The model under review builds one solid part; all positions refer to its coordinate system, in mm. A direction names the side the tool comes from. Give positions to 0.01 mm unless a question says otherwise; leave off trailing zeros. Write each question's results on one line, items separated by ' | '. Start each with the question number.
Q1. Machinability: for faces 5 (the face through (321, 11, -652.571)), 6 (the face through (321, 4, -649.396)), 7 (the face through (321, 24, -652.571)), 8 (the face through (318.96, 7, -681)), 9 (the face through (321, -0.32, -651)), which of the approach directions +Z, -Z, +X, -X, +Y, -Y give a long, thin tool a straight path to every point of the face, cutting with its end or side? Answer none if there is none.
Q2. Insertion check: pin 1 Ø1.6 at (x, z) = (320.5, -651.5) entering from +Y; pin 2 Ø1.1 at (x, y) = (321, 24) entering from +Z; pin 3 Ø1 at (x, z) = (320, -651) entering from -Y. Each pin has a flat end and moves straight along its axis. Give the tip position at first contact, or say it passes through.
Q3. Wall thickness on L1, parallel to Y at x = 320.15, z = -671; L2, parallel to Y at x = 320.15, z = -740: over which ranges is each line inside the solid? List them lowest first. Write a range as [from, to].
Q4. Mouldability with a two-part tool opening along Y and no side actions: class faces 1 (the face through (321, 13.65, -651)), 2 (the face through (321, -9, -764.915)), 3 (the face through (321, 22.54, -651)), 4 (the face through (321, 8.57, -651)) as released by +Y, released by -Y, zero draft, split by the parting line, or undercut.
from build123d import *

# Parameters (mm, degrees)
BOSS_EXTRUDE1_DEPTH = 3.175
CUT_EXTRUDE1_DEPTH  = 3.175
SKETCH3_W           = 3.175
SKETCH3_H           = 8.89
BOSS_EXTRUDE3_DEPTH = 3.175


with BuildPart() as part:
    # Sketch1 → Boss-Extrude1 (new body)
    with BuildSketch(Plane(origin=(322.1355, 0, 0), x_dir=(0, 0, -1), z_dir=(1, 0, 0))):
        with BuildLine():
            Line((652.571489798, 25.444691841), (652.571489798, -2.239853871))
            add(Edge.make_bspline(
                [(652.571489798, -2.239853871), (659.535508053, -2.166526792), (666.500386762, -2.172540218), (679.343468905, -2.343824355), (685.222739923, -2.485063976), (696.978954297, -2.909271923), (702.85456416, -3.191578316), (714.592323323, -3.919191383), (720.455505411, -4.364295636), (729.239801176, -5.181453913), (732.167256327, -5.479520855), (738.010202726, -6.135780349), (740.925935315, -6.494041299), (749.652482821, -7.677212837), (755.443511526, -8.605976907), (762.435970423, -9.996546686), (763.676377356, -10.253772029), (764.914772229, -10.521558234)],
                knots=[0.775497337, 0.775497337, 0.775497337, 0.775497337, 0.8125, 0.8125, 0.84375, 0.84375, 0.875, 0.875, 0.90625, 0.90625, 0.921875, 0.921875, 0.9375, 0.9375, 0.96875, 0.96875, 0.975501731, 0.975501731, 0.975501731, 0.975501731], degree=3))
            Line((764.914772229, -10.521558234), (764.914772229, -7.95557204))
            add(Edge.make_bspline(
                [(764.914772229, -7.95557204), (762.592495307, -6.961678807), (760.248039666, -6.021012379), (755.381001417, -4.157972035), (752.855549055, -3.242485253), (747.781003843, -1.468246605), (745.231905095, -0.60950889), (737.561144422, 1.91039187), (732.426406495, 3.521427695), (722.132037513, 6.655448313), (716.971446899, 8.176495188), (706.629978042, 11.149031985), (701.449248475, 12.601031652), (691.072587644, 15.45291135), (685.876480278, 16.853200873), (671.324621162, 20.706496058), (661.956512682, 23.109383547), (652.571489798, 25.444691841)],
                knots=[0.066165924, 0.066165924, 0.066165924, 0.066165924, 0.125, 0.125, 0.1875, 0.1875, 0.25, 0.25, 0.375, 0.375, 0.5, 0.5, 0.625, 0.625, 0.75, 0.75, 0.974669525, 0.974669525, 0.974669525, 0.974669525], degree=3))
        make_face()
    extrude(amount=-BOSS_EXTRUDE1_DEPTH)

    # Sketch2 → Cut-Extrude1 (cut)
    with BuildSketch(Plane.ZY.offset(-318.9605)):
        with BuildLine():
            Line((-649.396489798, 25.593288016), (-650.006698592, 28.058900562))
            add(Edge.make_bspline(
                [(-650.006698592, 28.058900562), (-660.51321247, 25.45866754), (-681.483078121, 20.093474052), (-707.597104431, 12.962630416), (-728.392690314, 6.856018534), (-743.920155817, 2.015224435), (-756.792636164, -2.379192874), (-766.929271878, -6.418935387), (-771.93415167, -8.70689296), (-774.395298331, -9.920762993)],
                knots=[0, 0, 0, 0, 0.25, 0.5, 0.625, 0.75, 0.875, 0.9375, 1, 1, 1, 1], degree=3))
            Line((-774.395298331, -9.920762993), (-773.271760863, -12.198758506))
            add(Edge.make_bspline(
                [(-649.396489798, 25.593288016), (-659.890092199, 22.996250426), (-670.36307543, 20.318524911), (-686.038941126, 16.170415704), (-691.258573313, 14.76557782), (-701.684945224, 11.905450655), (-706.891809106, 10.449729715), (-717.284977007, 7.471750728), (-722.471467171, 5.948931584), (-730.231305632, 3.598018149), (-732.814554878, 2.803107207), (-737.973199119, 1.186961553), (-740.549325052, 0.366607699), (-745.688759805, -1.3098747), (-748.250861629, -2.166692715), (-753.351930275, -3.936762543), (-755.890796198, -4.850260484), (-760.932732715, -6.76457283), (-763.436647752, -7.763327362), (-767.155712151, -9.351246242), (-768.389182844, -9.895718895), (-770.8414182, -11.020536997), (-772.060077224, -11.601140135), (-773.271760863, -12.198758506)],
                knots=[0, 0, 0, 0, 0.25, 0.25, 0.375, 0.375, 0.5, 0.5, 0.625, 0.625, 0.6875, 0.6875, 0.75, 0.75, 0.8125, 0.8125, 0.875, 0.875, 0.9375, 0.9375, 0.96875, 0.96875, 1, 1, 1, 1], degree=3))
        make_face()
    extrude(amount=-CUT_EXTRUDE1_DEPTH, mode=Mode.SUBTRACT)

    # Sketch3 → Boss-Extrude3 (add)
    with BuildSketch(Plane.XY.offset(-652.571489798)):
        with Locations((320.548, 18.094665768)):
            Rectangle(SKETCH3_W, SKETCH3_H)
        with Locations((320.548, 4.124665768)):
            Rectangle(SKETCH3_W, SKETCH3_H)
    extrude(amount=BOSS_EXTRUDE3_DEPTH)


solid = part.part
Output:
1) face 5: +Z, +X, -X | face 6: +Z, +X, -X, +Y, -Y | face 7: +Z, +X, -X, +Y | face 8: +Z, -Z, -X, +Y, -Y | face 9: +Z, +X, -X, -Y
2) pin 1: y = 22.54 | pin 2: z = -652.57 | pin 3: y = -0.32
3) L1: [-2.24, 20.12] | L2: [-6.39, 0.54]
4) face 1: undercut | face 2: zero draft | face 3: released by +Y | face 4: undercut
